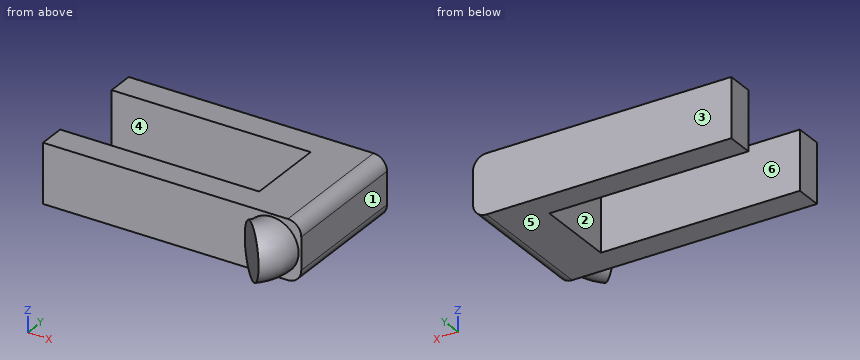
from build123d import *

# Parameters (mm, degrees)
F0_R     = 10
F2_ANGLE = 45
F3_W     = 22
F3_H     = 22
F3_R     = 10
F4_DEPTH = 50
F5_W     = 10
F5_H     = 22
F6_DEPTH = 74
F7_W     = 10
F7_H     = 22
F8_DEPTH = 74
F9_R     = 5


with BuildPart() as f2:
    # F0 (on Front) → F2 (revolve)
    with BuildSketch(Plane.XZ):
        Circle(F0_R)
    revolve(axis=Axis((-10.0093111396, 0, -0.720274169), (0, 0, -1)), revolution_arc=F2_ANGLE)

    # F3 (on face) → F4 (join)
    with BuildSketch(Plane(origin=(0, 0, 0), x_dir=(-1, 0, 0), z_dir=(0, 1, 0))):
        Rectangle(F3_W, F3_H)
        Circle(F3_R, mode=Mode.SUBTRACT)
        Circle(F3_R)
    extrude(amount=F4_DEPTH)

    # F5 (on face) → F6 (join)
    with BuildSketch(Plane(origin=(-11, 0, 0), x_dir=(0, -1, 0), z_dir=(-1, 0, 0))):
        with Locations((-5, 0)):
            Rectangle(F5_W, F5_H)
    extrude(amount=F6_DEPTH)

    # F7 (on face) → F8 (join)
    with BuildSketch(Plane(origin=(-11, 0, 0), x_dir=(0, -1, 0), z_dir=(-1, 0, 0))):
        with Locations((-45, 0)):
            Rectangle(F7_W, F7_H)
    extrude(amount=F8_DEPTH)

    # F9
    f9_edges = [f2.edges().sort_by_distance(p)[0] for p in [
        (11, 25, -11),
        (11, 25, 11),
    ]]
    fillet(f9_edges, radius=F9_R)


solid = f2.part
Check sheet for the modelled part. Datum: model origin and axes. Units: mm. Face numbers are marked on the shaded views. A direction names the side the tool comes from. Round coordinates to 2 decimals unless told otherwise and drop trailing zeros. Order: outer loops, then holes, each group sorted by start corner. A loop starts at its lowest first (then second) coordinate and runs counter-clockwise, first axis right, second up.
(1) Scan lines: probe 1 along Y at (x, z) = (-48, 0.75); probe 2 along X at (y, z) = (27, -0.5); probe 3 along X at (y, z) = (2, 7). Record each from-to range of solid material in increasing order.
(2) Access from +Z, -Z, +X, -X, +Y, -Y to the whole of each face (thin tool, end or side, straight path). Record for the marked faces 1 and 2.
(3) Cross-section at A-A, the plane x = -13. Enter the section's corners in (y, z), and give its area (3 significant figures).
(4) Go/stop test with flat-tipped pins: P1, Ø1.5, axis at x = -22.5, z = -4, coming from the -Y side; P2, Ø12, axis at y = -2.5, z = 2.5, coming from the +X side; P3, Ø6.5, axis at y = 25, z = 1, coming from the -X side. Record where each tip stops, or that it passes through.
(5) Cross-section at C-C, the plane z = 4. Enter the section's corners in (x, y).
(6) Draft check along Y on the marked faces 3, 4, 5 and 6. Enter one of: pulls with the +Y half, pulls with the -Y half, needs draft (parallel to the pull), parting line crosses it, or undercut.
(7) Cross-section at D-D, the plane z = -9. Enter the section's corners in (x, y).
(8) Cross-section at B-B, the plane y = 33. Enter the section's corners in (x, z), and give its area (3 significant figures).
Check sheet entries:
1. probe 1: y = 0 to 10, 40 to 50
1. probe 2: x = -11 to 11
1. probe 3: x = -85 to 10.9
2. face 1: +Z, -Z, +X, +Y, -Y
2. face 2: +Z, -Z, -X
3. outline: (0, -11) - (10, -11) - (10, 11) - (0, 11) - close; (40, -11) - (50, -11) - (50, 11) - (40, 11) - close
3. area: 440 mm2
4. P1: stops at y = 0
4. P2: stops at x = 11
4. P3: stops at x = -11
5. outline: (-85, 0) - (-9.17, 0) arc R0.84 cw to (-9.41, -0.6) - (3.55, -13.56) arc R19.17 ccw to (9.17, 0) - (11, 0) - (11, 50) - (-85, 50) - (-85, 40) - (-11, 40) - (-11, 10) - (-85, 10) - close
6. face 3: pulls with the +Y half
6. face 4: undercut
6. face 5: needs draft
6. face 6: undercut
7. outline: (-85, 0) - (-4.36, 0) arc R5.65 cw to (-6.01, -4) - (0.15, -10.16) arc R14.37 ccw to (4.36, 0) - (10, 0) - (10, 50) - (-85, 50) - (-85, 40) - (-11, 40) - (-11, 10) - (-85, 10) - close
8. outline: (-11, -11) - (6, -11) arc R5 ccw to (11, -6) - (11, 6) arc R5 ccw to (6, 11) - (-11, 11) - close
8. area: 473 mm2
